from build123d import *

# Parameters (mm, degrees)
F0_R     = 50.8
F0_R_2   = 24.4152864436
F0_R_3   = 14.7083689978
F0_R_4   = 9.8191512815
F1_DEPTH = 12.7
F2_R     = 24.9173840561
F2_R_2   = 19.2210647441
F3_DEPTH = 50.8
F7_R     = 19.05
F7_R_2   = 15.875
F8_DEPTH = 6.35
F9_R     = 1.524
F10_R    = 2.54


with BuildPart() as f1:
    # F0 (on Front) → F1 (new body)
    with BuildSketch(Plane.XZ):
        Circle(F0_R)
        with BuildLine():
            ThreePointArc((4.8233222323, -38.1), (-0.1527303768, -42.9209035241), (-4.8136498253, -37.7946924231))
            ThreePointArc((-4.8136498253, -37.7946924231), (-18.3999542583, -33.3624292175), (-29.3974979615, -24.2362768099))
            ThreePointArc((-29.3974979615, -24.2362768099), (-36.9844148106, -23.5242456402), (-34.4130307135, -16.3509423923))
            ThreePointArc((-34.4130307135, -16.3509423923), (-38.0164573377, -2.5217001197), (-36.2712015434, 11.6623298959))
            ThreePointArc((-36.2712015434, 11.6623298959), (-38.8755747903, 18.1961885071), (-32.1899666774, 20.3817576599))
            ThreePointArc((-32.1899666774, 20.3817576599), (-21.7323643265, 31.2939984786), (-7.8547610469, 37.2815333496))
            ThreePointArc((-7.8547610469, 37.2815333496), (-3.6092020095, 40.8787866416), (1.2009713639, 38.0810670515))
            ThreePointArc((1.2009713639, 38.0810670515), (17.0828495941, 34.0556346255), (29.8056914767, 23.7324831317))
            ThreePointArc((29.8056914767, 23.7324831317), (33.1670019723, 22.2933561664), (34.5529237527, 18.9097611124))
            ThreePointArc((34.5529237527, 18.9097611124), (34.4459537327, 17.8995833234), (34.1297883633, 16.9342123016))
            ThreePointArc((34.1297883633, 16.9342123016), (37.0941702741, 8.6966965958), (38.1, 0))
            ThreePointArc((38.1, 0), (37.3167165393, -7.6858744934), (34.9990726127, -15.0557270251))
            ThreePointArc((34.9990726126, -15.0557270251), (35.8497747537, -16.5146045982), (36.1454234548, -18.1773161641))
            ThreePointArc((36.1454234548, -18.1773161641), (34.4035372294, -21.8880020161), (30.4360020939, -22.9185465626))
            ThreePointArc((30.4360020939, -22.9185465626), (19.1300658394, -32.949212145), (4.8136498253, -37.7946924231))
            ThreePointArc((4.8136498253, -37.7946924231), (4.8209035241, -37.9472696232), (4.8233222323, -38.1))
        make_face(mode=Mode.SUBTRACT)
        with BuildLine():
            Line((-28.6378667765, -23.1658492328), (-4.2767341482, -35.8697573266))
            ThreePointArc((-4.2767341482, -35.8697573266), (-0.2069202623, -33.2811182457), (4.0698138859, -35.5113609191))
            Line((4.0698138859, -35.5113609191), (27.2522873366, -20.765955245))
            ThreePointArc((27.2522873366, -20.765955245), (27.0453670743, -15.9470734907), (31.1151809602, -13.3584344098))
            Line((31.1151809602, -13.3584344098), (29.9365217826, 14.0908793581))
            ThreePointArc((29.9365217826, 14.0908793581), (25.6597876344, 16.3211220315), (25.4528673721, 21.1400037858))
            Line((25.4528673721, 21.1400037858), (1.0917347439, 33.8439118796))
            ThreePointArc((1.0917347439, 33.8439118796), (-2.978079142, 31.2552727988), (-7.2548132903, 33.4855154722))
            Line((-7.2548132903, 33.4855154722), (-30.437286741, 18.7401097981))
            ThreePointArc((-30.437286741, 18.7401097981), (-29.8759851482, 17.4995088397), (-29.6837783945, 16.1514707172))
            ThreePointArc((-29.6837783945, 16.1514707172), (-31.0241076281, 12.814826126), (-34.3001803645, 11.3325889629))
            Line((-34.3001803645, 11.3325889629), (-33.121521187, -16.116724805))
            ThreePointArc((-33.121521187, -16.116724805), (-29.5779563335, -17.4526135606), (-28.0912786923, -20.9356065593))
            ThreePointArc((-28.0912786923, -20.9356065593), (-28.229918211, -22.0837290393), (-28.6378667765, -23.1658492328))
        make_face()
        Circle(F0_R_2, mode=Mode.SUBTRACT)
        Circle(F0_R_2)
        Circle(F0_R_3, mode=Mode.SUBTRACT)
        Circle(F0_R_3)
        Circle(F0_R_4, mode=Mode.SUBTRACT)
        with BuildLine():
            Line((29.9365217826, 14.0908793581), (31.1151809602, -13.3584344098))
            ThreePointArc((31.1151809602, -13.3584344098), (33.2535551471, -13.757596366), (34.9990726126, -15.0557270251))
            ThreePointArc((34.9990726127, -15.0557270251), (37.3167165393, -7.6858744934), (38.1, 0))
            ThreePointArc((38.1, 0), (37.0941702741, 8.6966965958), (34.1297883633, 16.9342123016))
            ThreePointArc((34.1297883633, 16.9342123016), (32.4365360461, 14.91765104), (29.9365217826, 14.0908793581))
        make_face()
        with BuildLine():
            Line((27.2522873366, -20.765955245), (4.0698138859, -35.5113609191))
            ThreePointArc((4.0698138859, -35.5113609191), (4.5861075616, -36.6059937113), (4.8136498253, -37.7946924231))
            ThreePointArc((4.8136498253, -37.7946924231), (19.1300658394, -32.949212145), (30.4360020939, -22.9185465626))
            ThreePointArc((30.4360020939, -22.9185465626), (28.6204941458, -22.1730334414), (27.2522873366, -20.765955245))
        make_face()
        with BuildLine():
            ThreePointArc((-4.8136498253, -37.7946924231), (-4.6459782584, -36.8041128988), (-4.2767341482, -35.8697573266))
            Line((-4.2767341482, -35.8697573266), (-28.6378667765, -23.1658492328))
            ThreePointArc((-28.6378667765, -23.1658492328), (-28.98110019, -23.7270236417), (-29.3974979615, -24.2362768099))
            ThreePointArc((-29.3974979615, -24.2362768099), (-18.3999542583, -33.3624292175), (-4.8136498253, -37.7946924231))
        make_face()
        with BuildLine():
            ThreePointArc((-36.2712015434, 11.6623298959), (-38.0164573377, -2.5217001197), (-34.4130307135, -16.3509423923))
            ThreePointArc((-34.4130307135, -16.3509423923), (-33.7752804055, -16.1896958787), (-33.121521187, -16.116724805))
            Line((-33.121521187, -16.116724805), (-34.3001803645, 11.3325889629))
            ThreePointArc((-34.3001803645, 11.3325889629), (-35.3029556188, 11.3942601702), (-36.2712015434, 11.6623298959))
        make_face()
        with BuildLine():
            ThreePointArc((-7.8547610469, 37.2815333496), (-21.7323643265, 31.2939984786), (-32.1899666774, 20.3817576599))
            ThreePointArc((-32.1899666774, 20.3817576599), (-31.209824844, 19.6717561841), (-30.437286741, 18.7401097981))
            Line((-30.437286741, 18.7401097981), (-7.2548132903, 33.4855154722))
            ThreePointArc((-7.2548132903, 33.4855154722), (-7.9491869569, 35.3211908614), (-7.8547610469, 37.2815333496))
        make_face()
        with BuildLine():
            Line((1.0917347439, 33.8439118796), (25.4528673721, 21.1400037858))
            ThreePointArc((25.4528673721, 21.1400037858), (27.2614868155, 23.0537745246), (29.8056914767, 23.7324831317))
            ThreePointArc((29.8056914767, 23.7324831317), (17.0828495941, 34.0556346255), (1.2009713639, 38.0810670515))
            ThreePointArc((1.2009713639, 38.0810670515), (1.5277167803, 37.1011616221), (1.638322828, 36.0741545531))
            ThreePointArc((1.638322828, 36.0741545531), (1.4996833093, 34.9260320731), (1.0917347439, 33.8439118796))
        make_face()
    extrude(amount=F1_DEPTH)

    # F2 (on Front) → F3 (join)
    with BuildSketch(Plane.XZ):
        Circle(F2_R)
        Circle(F2_R_2, mode=Mode.SUBTRACT)
    extrude(amount=-F3_DEPTH)

    # F5 (on Right) → F6 (revolve)
    with BuildSketch(Plane.YZ):
        Polygon((50.8, -19.1665568061), (0, -6.4665568061), (0, -19.1665568061), align=None)
    revolve(axis=Axis((0, 25.7261283696, 0), (0, -1, 0)))

    # F7 (on face) → F8 (join)
    with BuildSketch(Plane.XZ.offset(12.7)):
        Circle(F7_R)
        Circle(F7_R_2, mode=Mode.SUBTRACT)
    extrude(amount=F8_DEPTH)

    # F9
    f9_edges = [f1.edges().sort_by_distance(p)[0] for p in [
        (-19.05, -19.05, 0),
        (-15.875, -19.05, 0),
    ]]
    fillet(f9_edges, radius=F9_R)

    # F10
    f10_edges = [f1.edges().sort_by_distance(p)[0] for p in [
        (-50.8, -12.7, 0),
        (-50.8, 0, 0),
    ]]
    fillet(f10_edges, radius=F10_R)


solid = f1.part
Work out the finished part from the listing and answer in its coordinate system (mm). A direction names the side the tool comes from. Give positions to 0.01 mm unless a question says otherwise; leave off trailing zeros. Loops run counter-clockwise (first coordinate to the right, second up) from the corner with the lowest first, then second, coordinate; pieces in that order, holes last. Notation, with made-up numbers: (0, -18.5) -> (33, -18.5) arc R26 cw to (33, -4.5) -> close; hole circle Ø1 at (-25, -37). An arc over 180 degrees is marked (long way). Use a Markdown table: item, result. Add a question column.
1) The part is cut by section A-A, the plane y = 16. Determine the outline of the cut face in (x, z).
2) The part is cut by section B-B, the plane y = 33. Determine the outline of the cut face in (x, z).
3) Each of these flat-tipped pins is pushed along its axis until it touches: P1, Ø4, axis at x = 33.5, z = 16.5, coming from the -Y side; P2, Ø5, axis at x = -17.5, y = 19.5, coming from the -Z side; P3, Ø19, axis at x = 0, z = 0, coming from the -Y side. Where does it stop, or does it pass through?
4) Consider line 1 along Z through (x, y) = (0, -4.5); line 2 along Y through (x, z) = (-33.5, 9); line 3 along Z through (x, y) = (0, -2). Determine where each line is inside the solid, lowest interval first.
5) For a pull along Z with two mould halves and no side action, classify faces 4 (the flat face through (21, 0, -21)), 5 (the cylindrical face through (-1.278, -6.261, 9.736)), 6 (the cylindrical face through (-11.012, -6.297, -49.592)), 7 (the flat face through (-2, 0, 6.4)) as +Z half, -Z half, draft (parallel to the pull), parting line (faces both ways), or undercut.
6) Which of the six approach directions +Z, -Z, +X, -X, +Y, -Y give full straight-line access (tool end or side, diameter ignored) to faces 1 (the flat face through (13, 50.8, -15)), 2 (the flat face through (6.8, -12.7, 7.3)), 3 (the cylindrical face through (-3.244, 25.044, 24.705))?
Reported:
| question | item | result |
|---|---|---|
| 1 | outline | circle Ø49.83 at (0, 0); circle Ø38.33 at (0, 0); hole circle Ø38.44 at (0, 0); hole circle Ø20.93 at (0, 0) |
| 2 | outline | circle Ø49.83 at (0, 0); circle Ø38.33 at (0, 0); hole circle Ø38.44 at (0, 0); hole circle Ø29.43 at (0, 0) |
| 3 | P1 | stops at y = -12.7 |
| 3 | P2 | stops at z = -19.9 |
| 3 | P3 | stops at y = 0 |
| 4 | line 1 | z = -50.8 to -42.92, -33.28 to -9.82, 9.82 to 32.45, 39.7 to 50.8 |
| 4 | line 2 | y = -12.7 to 0 |
| 4 | line 3 | z = -50.74 to -42.92, -33.28 to -9.82, 9.82 to 32.45, 39.7 to 50.74 |
| 5 | face 4 | draft |
| 5 | face 5 | undercut |
| 5 | face 6 | parting line |
| 5 | face 7 | undercut |
| 6 | face 1 | +Z, -Z, +X, -X, +Y |
| 6 | face 2 | -Y |
| 6 | face 3 | +Y |
